Print and shaded views of the part. All mm, measured from the part's lowest x, y and z. A direction names the side the tool comes from. Give positions to 0.01 mm unless a question says otherwise; leave off trailing zeros. Loops run counter-clockwise (first coordinate to the right, second up) from the corner with the lowest first, then second, coordinate; pieces in that order, holes last. Notation, with made-up numbers: M 31.5,84 L 66.5,84 A27 cw 66.5,101 Z; hole C 17,52.5 d1. An arc over 180 degrees is marked long. Answer as CSV lines item,"result".
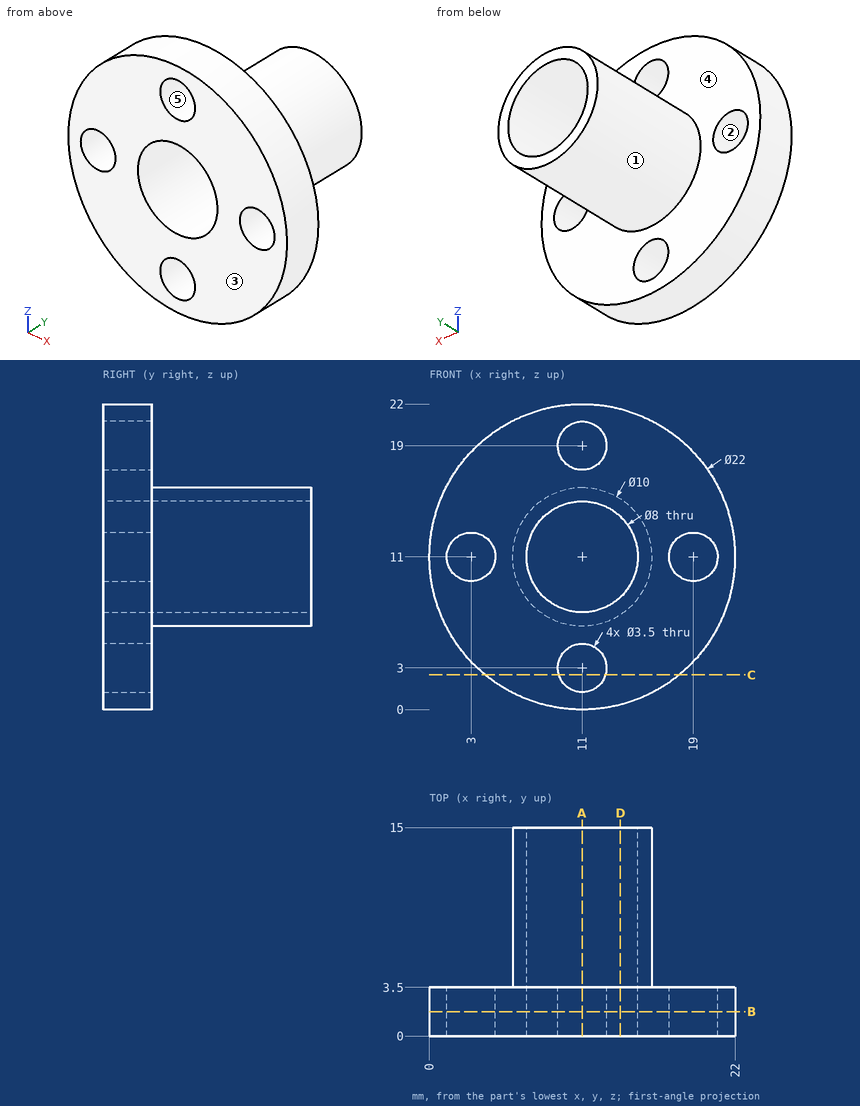
Q1. Wall check: line 1 (X direction, y = 1.25, z = 11); line 2 (X direction, y = 11.75, z = 11); line 3 (Y direction, x = 6.5, z = 17.5). Give the ranges that are in metal, low to high. Write a range as [from, to].
Solution:
line 1,"x = [0, 1.25], [4.75, 7], [15, 17.25], [20.75, 22]"
line 2,"x = [6, 7], [15, 16]"
line 3,"y = [0, 3.5]"
Q2. Which spindle directions (+Z, -Z, +X, -X, +Y, -Y) get a long thin tool onto all of the face, cutting with end or side? Do the marked faces 4 and 5. Say none if no direction does.
Solution:
face 4,"+Y"
face 5,"+Y, -Y"
Q3. Pin check, flat tips, straight feed: P1, Ø13, axis at x = 11, z = 11, coming from the -Y side; P2, Ø1.5, axis at x = 19.5, z = 12, coming from the +Y side; P3, Ø5, axis at y = 7, z = 4, coming from the -X side; P4, Ø3, axis at y = 8.5, z = 8, coming from the +X side. Stop position of each tip, or through.
Solution:
P1,"stops at y = 0"
P2,"stops at y = 3.5"
P3,"stops at x = 8.82"
P4,"stops at x = 15.77"
Q4. Mould opens along Z. For the marked faces 1, 2 and 3 say: released by +Z, released by -Z, zero draft, split by the parting line, or undercut.
Solution:
face 1,"split by the parting line"
face 2,"undercut"
face 3,"zero draft"
Q5. Cut at C-C (z = 2.5). Write the cut outline in (x, y).
Solution:
outline,"M 4.02,0 L 9.32,0 L 9.32,3.5 L 4.02,3.5 Z; M 12.68,0 L 17.98,0 L 17.98,3.5 L 12.68,3.5 Z"
Q6. Cut at A-A (x = 11). Write the cut outline in (y, z), and give its area (3 significant figures).
Solution:
outline,"M 0,0 L 3.5,0 L 3.5,1.25 L 0,1.25 Z; M 0,4.75 L 3.5,4.75 L 3.5,6 L 15,6 L 15,7 L 0,7 Z; M 0,15 L 15,15 L 15,16 L 3.5,16 L 3.5,17.25 L 0,17.25 Z; M 0,20.75 L 3.5,20.75 L 3.5,22 L 0,22 Z"
area,"47.5 mm²"
Q7. Cut at D-D (x = 13.75). Write the cut outline in (y, z).
Solution:
outline,"M 0,0.35 L 3.5,0.35 L 3.5,6.82 L 15,6.82 L 15,8.1 L 0,8.1 Z; M 0,13.9 L 15,13.9 L 15,15.18 L 3.5,15.18 L 3.5,21.65 L 0,21.65 Z"
Q8. Cut at B-B (y = 1.75). Write the cut outline in (x, z), and give its area (3 significant figures).
Solution:
outline,"C 11,11 d22; hole C 3,11 d3.5; hole C 11,11 d8; hole C 11,3 d3.5; hole C 11,19 d3.5; hole C 19,11 d3.5"
area,"291 mm²"
